Geometry: final body of the model. Coordinates: model frame, mm. A direction names the side the tool comes from. Coordinates: 2 decimals unless noted, no trailing zeros. Order: outer loops, then holes, each group sorted by start corner. A loop starts at its lowest first (then second) coordinate and runs counter-clockwise, first axis right, second up. Notation, with made-up numbers: (-33.75, 35.25) -> (-22.75, 35.25) arc R23 ccw to (-22.75, 51.25) -> close; hole circle Ø3 at (56, 63.5). An arc over 180 degrees is marked (long way). Use one line per item in the form item = value.
Autodesk Inventor part; units mm, degrees
ref_plane "YZ Plane" through (0, 0, 0) normal (1, 0, 0) x (0, 1, 0)
ref_plane "XZ Plane" through (0, 0, 0) normal (0, 1, 0) x (-1, 0, 0)
ref_plane "XY Plane" through (0, 0, 0) normal (0, 0, 1) x (1, 0, 0)
sketch "Sketch1" plane through (0, 0, 0) normal (1, 0, 0) x (0, 1, 0)
  circle A0 centre (0, 0) radius 2.4765
  dimension "d1" = 4.953
extrude "Extrusion1" add sketch "Sketch1" along normal blind 3.048
sketch "Sketch2" plane through (3.048, 0, 0) normal (1, 0, 0) x (0, 0, -1)
  circle A0 centre (0, 0) radius 2.4765
  circle A1 centre (0, 0) radius 1.397
  dimension "d5" = 2.794
extrude "Extrusion2" add sketch "Sketch2" along normal blind 13.081 contours A1
sketch "Sketch3" plane through (16.129, 0, 0) normal (1, 0, 0) x (0, 0, -1)
  circle A0 centre (0, 0) radius 1.397
  circle A1 centre (0, 0) radius 0.8128
  dimension "d8" = 1.6256
extrude "Extrusion3" add sketch "Sketch3" along normal blind 3.9116 contours A1
chamfer "Chamfer1" distance 0.508 angle 45 1 edges at (16.129, 0, 0.8128)
thread "Thread1"
sketch "Sketch4" plane through (0, 0, 0) normal (-1, 0, 0) x (0, 0, 1)
  circle A0 centre (0, 0) radius 2.4765
  line L0 (-2.4765, 0.5207) -> (2.4765, 0.5207)
  line L1 (2.4765, 0.5207) -> (2.4765, -0.5207)
  line L2 (2.4765, -0.5207) -> (-2.4765, -0.5207)
  line L3 (-2.4765, -0.5207) -> (-2.4765, 0.5207)
  dimension "d16" = 1.0414
  dimension "d18" = 0.5207
extrude "Extrusion4" cut sketch "Sketch4" against normal blind 0.7366 contours A0 L2 L0 | L1 L2 A0 | A0 L0 L1 | A0 L3 L0 | L2 L3 A0
equation "\"d18\" = 0.5 * d16"
properties part number "Air Adjuster"
1) Section B-B, the plane z = 0. Output: boundary loops of the cut face in (x, y), and give its area (3 significant figures).
Results found:
outline = (0, -2.48) -> (3.05, -2.48) -> (3.05, -1.4) -> (16.13, -1.4) -> (16.13, -1.32) -> (16.64, -0.81) -> (20.04, -0.81) -> (20.04, 0.81) -> (16.64, 0.81) -> (16.13, 1.32) -> (16.13, 1.4) -> (3.05, 1.4) -> (3.05, 2.48) -> (0, 2.48) -> (0, 0.52) -> (0.74, 0.52) -> (0.74, -0.52) -> (0, -0.52) -> close
area = 57.5 mm2
2) Material intervals for probe 1 along X at (y, z) = (-1.2, 1); probe 2 along X at (y, z) = (-0.4, 0.15); probe 3 along Z at (x, y) = (7.75, -0.05), sorted ascending. Write a range as from..to.
Results found:
probe_1 = 0..3.05
probe_2 = 0.74..20.04
probe_3 = -1.4..1.4
3) Section C-C, the plane x = 12. Output: boundary loops of the cut face in (y, z), and give its area (3 significant figures).
Results found:
outline = circle Ø2.79 at (0, 0)
area = 6.13 mm2
4) Section A-A, the plane y = 0. Output: boundary loops of the cut face in (x, z), and give its area (3 significant figures).
Results found:
outline = (0.74, -2.48) -> (3.05, -2.48) -> (3.05, -1.4) -> (16.13, -1.4) -> (16.13, -1.32) -> (16.64, -0.81) -> (20.04, -0.81) -> (20.04, 0.81) -> (16.64, 0.81) -> (16.13, 1.32) -> (16.13, 1.4) -> (3.05, 1.4) -> (3.05, 2.48) -> (0.74, 2.48) -> close
area = 54.6 mm2
5) Contact query for flat-ended pins moving along their axis: P1, Ø1, axis at x = 6, z = -1.5, coming from the +Y side; P2, Ø1.5, axis at x = 14, y = 0, coming from the +Z side; P3, Ø1, axis at x = 12.5, z = 0, coming from the -Y side. Output: stop coordinate, or through.
Results found:
P1 = 0.98
P2 = 1.4
P3 = -1.4
6) Section D-D, the plane z = -1.85. Output: boundary loops of the cut face in (x, y), and give its area (3 significant figures).
Results found:
outline = (0, -1.65) -> (3.05, -1.65) -> (3.05, 1.65) -> (0, 1.65) -> (0, 0.52) -> (0.74, 0.52) -> (0.74, -0.52) -> (0, -0.52) -> close
area = 9.27 mm2
7) Access query for faces 1 (the cylindrical face through (9.5, 0.85, 1.11)), 2 (the flat face through (0.737, 0, 0)), 3 (the flat face through (0, 1, 0)). Directions: +Z, -Z, +X, -X, +Y, -Y. A direction counts if a zero-diameter tool reaches every point of the face in a straight line with its end or side. Return the directions, or none.
Results found:
face_1 = +X
face_2 = +Z, -Z, -X
face_3 = +Z, -Z, -X, +Y, -Y
